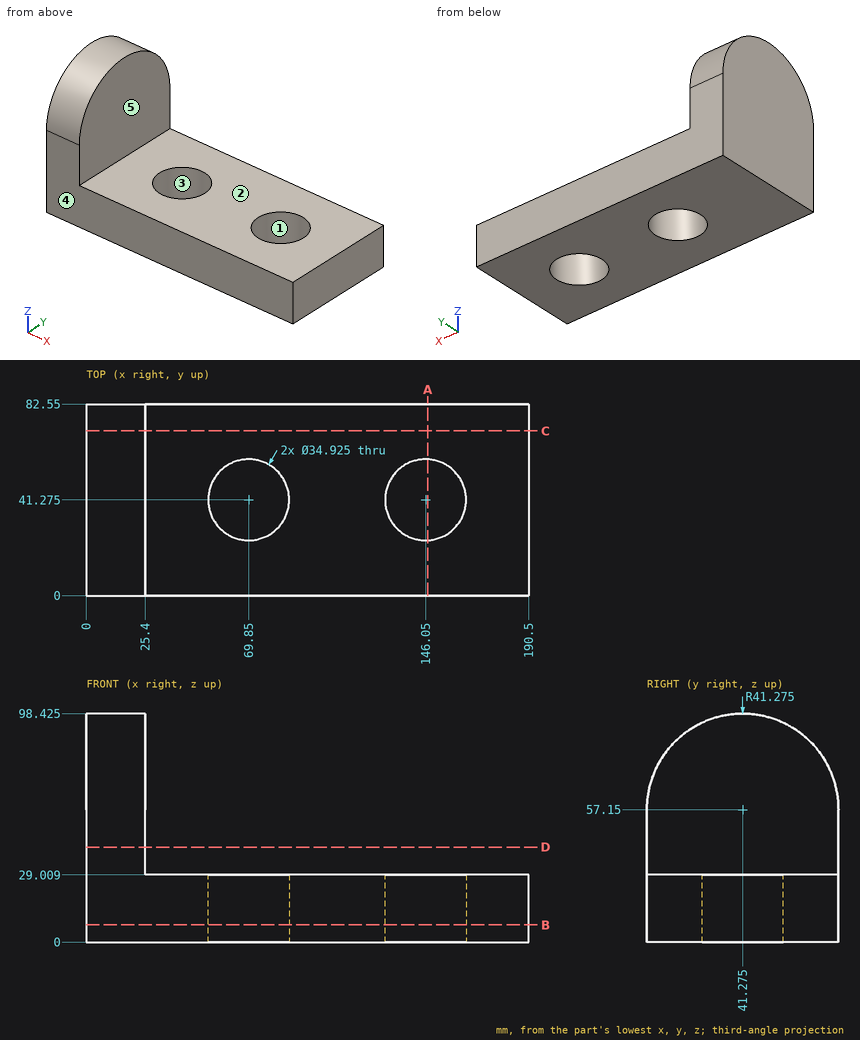
Job drawing, mm, ordinate dimensions from the low corner. One solid piece. A direction names the side the tool comes from. Give positions to 0.01 mm unless a question says otherwise; leave off trailing zeros. Write each loop counter-clockwise with the first axis right and the second up, starting at its lowest first coordinate (ties: lowest second). Pieces come first, ordered by that corner, then holes. Notation, with made-up numbers: (39.5, 54) - (59.5, 54) arc R17 ccw to (59.5, 81) - close; hole circle Ø3 at (-8.5, -2.75). An arc over 180 degrees is marked (long way). Answer as CSV lines item,"result".
1. Pin check, flat tips, straight feed: pin 1 (1.5 mm diameter, centred on y = 47.5, z = 40, fed in from -X); pin 2 (25 mm diameter, centred on x = 76.5, y = 32.5, fed in from +Z); pin 3 (5 mm diameter, centred on x = 23, z = 66.5, fed in from +Y); pin 4 (5 mm diameter, centred on y = 18.5, z = 34.5, fed in from +X). Stop position of each tip, or through.
Responses:
pin 1,"stops at x = 0"
pin 2,"stops at z = 29.01"
pin 3,"stops at y = 81.98"
pin 4,"stops at x = 25.4"
2. Two-plate mould, pull along Y, no slides. Class the marked faces 3, 4 and 5: +Y half, -Y half, draft (parallel to the pull), parting line (faces both ways), or undercut.
Responses:
face 3,"undercut"
face 4,"-Y half"
face 5,"draft"
3. Band-saw the part on C-C (y = 71). Write the cut outline in (x, z), and give its area (3 significant figures).
Responses:
outline,"(0, 0) - (190.5, 0) - (190.5, 29.01) - (25.4, 29.01) - (25.4, 85.79) - (0, 85.79) - close"
area,"6,970 mm2"
4. Band-saw the part on B-B (z = 7.5). Count the separate pieces of the cut face and the enclosed holes in it, and give its area (3 significant figures).
Responses:
separate pieces,"1"
enclosed holes,"2"
area,"13,800 mm2"
5. Drill centre lines: L1, parallel to Y at x = 69, z = 20; L2, parallel to X at y = 55, z = 7.5 (1 decimal); L3, parallel to Z at x = 115, y = 11. Where is each one in solid material? Low to high. Write a range as [from, to].
Responses:
L1,"y = [0, 23.83], [58.72, 82.55]"
L2,"x = [0, 59.1], [80.6, 135.3], [156.8, 190.5]"
L3,"z = [0, 29.01]"
6. 3-axis set-ups, long thin cutter, end or side, ignore diameter. For the marked faces 1 and 2: which of +Z, -Z, +X, -X, +Y, -Y reach the whole face in a straight line?
Responses:
face 1,"+Z, -Z"
face 2,"+Z, +X, +Y, -Y"
7. Band-saw the part on D-D (z = 41). Write the cut outline in (x, y).
Responses:
outline,"(0, 0) - (25.4, 0) - (25.4, 82.55) - (0, 82.55) - close"
8. Band-saw the part on A-A (x = 147). Write the cut outline in (y, z).
Responses:
outline,"(0, 0) - (23.84, 0) - (23.84, 29.01) - (0, 29.01) - close; (58.71, 0) - (82.55, 0) - (82.55, 29.01) - (58.71, 29.01) - close"
